Here's how the part is built. I have some questions about the finished solid (model axes, mm). Face numbers are marked on the shaded views. A direction names the side the tool comes from. Round coordinates to 2 decimals unless told otherwise and drop trailing zeros. Write each loop counter-clockwise with the first axis right and the second up, starting at its lowest first coordinate (ties: lowest second). Pieces come first, ordered by that corner, then holes. Notation, with made-up numbers: (3, 27.5) - (52, 27.5) arc R36 ccw to (52, 64.5) - close; hole circle Ø1 at (58, -15). An arc over 180 degrees is marked (long way). Write item = value, one per line. Start each with the question number.
Item 1: Thinking about a two-plate mould opening in Z: for the marked faces 3, 4 and 5, which applies, pulls with the +Z half, pulls with the -Z half, needs draft (parallel to the pull), parting line crosses it, or undercut?
Item 2: Which directions (+Z, -Z, +X, -X, +Y, -Y) give clear straight access to the entire face, cutting with the end or side of a thin tool? Please do the marked faces 1 and 2.
Item 3: If we section it at D-D (x = 64): Please give me the cut outline in (y, z), and give its area (3 significant figures).
Item 4: If we section it at A-A (y = 57): Please give me the cut outline in (x, z), and give its area (3 significant figures).
Item 5: For P1, Ø4, axis at x = -69.3, z = -81.8, coming from the +Y side; P2, Ø1.5, axis at x = -69.5, z = 81, coming from the -Y side; P3, Ø2, axis at x = 12, y = 74, coming from the +Z side, each with a flat end and sliding along its axis, tell me the tip position at first contact or that it passes through.
Item 6: If we section it at B-B (x = -69.3): Please give me the cut outline in (y, z).
Item 7: If I drill on line 1 along Z through (x, y) = (-69.3, 2); line 2 along X through (y, z) = (78, -24.5); line 3 along Z through (x, y) = (0, 63), over which ranges is the centre line in solid material (lowest first)? Write a range as [from, to].
Item 8: If we section it at C-C (z = -24.5): Please give me the cut outline in (x, y), and give its area (3 significant figures).
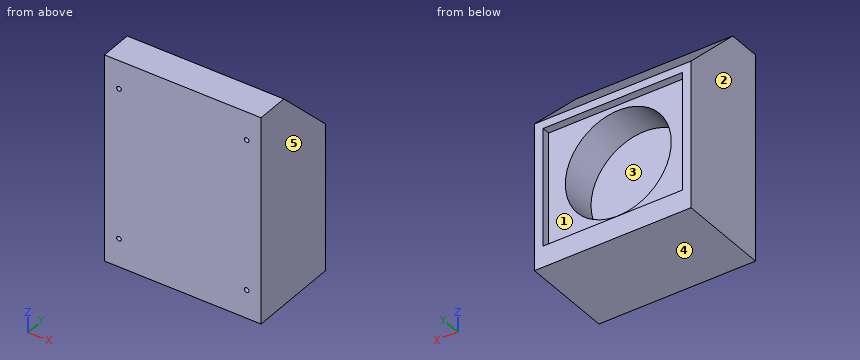
Autodesk Inventor part; units mm, degrees
ref_plane "YZ Plane" through (0, 0, 0) normal (1, 0, 0) x (0, 1, 0)
ref_plane "XZ Plane" through (0, 0, 0) normal (0, 1, 0) x (-1, 0, 0)
ref_plane "XY Plane" through (0, 0, 0) normal (0, 0, 1) x (1, 0, 0)
sketch "Sketch1" plane through (0, 0, 0) normal (0, 1, 0) x (-1, 0, 0)
  line L0 (-85, 112.5) -> (85, 112.5)
  line L1 (85, 112.5) -> (85, -112.5)
  line L2 (85, -112.5) -> (-85, -112.5)
  line L3 (-85, -112.5) -> (-85, 112.5)
  line L4 (-85, 112.5) -> (85, -112.5) construction
  line L5 (85, 112.5) -> (-85, -112.5) construction
  circle A0 centre (69.3, 81.8) radius 2.5
  circle A1 centre (69.3, -81.8) radius 2.5
  circle A2 centre (-69.3, -81.8) radius 2.5
  circle A3 centre (-69.3, 81.8) radius 2.5
  line L6 (69.3, 81.8) -> (-69.3, 81.8) construction
  line L7 (69.3, 81.8) -> (69.3, -81.8) construction
  line L8 (69.3, -81.8) -> (-69.3, -81.8) construction
  line L9 (69.3, 0) -> (0, 0) construction
  line L10 (0, 81.8) -> (0, 0) construction
  dimension "d2" = 170
  dimension "d3" = 225
  dimension "d9" = 163.6
  dimension "d10" = 5
  dimension "d11" = 138.6
extrude "Extrusion1" add sketch "Sketch1" along normal blind 100.5 contours L0 L1 L2 L3 | A0 | A1 | A2 | A3
extrude "Extrusion2" cut sketch "Sketch1" along normal blind 10 contours A0 | A1 | A2 | A3
chamfer "Chamfer1" distance 65 angle 45 1 edges at (0, 100.5, 112.5)
sketch "Sketch2" plane through (0, 100.5, 0) normal (0, 1, 0) x (1, 0, 0)
  line L0 (75.65, -38.8) -> (-75.65, -38.8)
  line L1 (-75.65, -38.8) -> (-75.65, 89.5)
  line L2 (-75.65, 89.5) -> (75.65, 89.5)
  line L3 (75.65, 89.5) -> (75.65, -38.8)
  line L4 (75.65, -38.8) -> (-75.65, 89.5) construction
  line L5 (-75.65, -38.8) -> (75.65, 89.5) construction
  line L6 (85, -47.5) -> (-85, -47.5)
  line L7 (85, -47.5) -> (85, 112.5)
  line L8 (85, 112.5) -> (-85, 112.5)
  line L9 (-85, 112.5) -> (-85, -47.5)
  line L10 (0, 89.5) -> (0, 112.5) construction
  circle A0 centre (0, 24.5) radius 57.5
  line L11 (0, 24.5) -> (0, 82) construction
  line L12 (0, 82) -> (0, 89.5) construction
  point P0 (0, 0)
  dimension "d21" = 115
  dimension "d18" = 151.3
  dimension "d19" = 128.3
  dimension "d20" = 23
  dimension "d22" = 7.5
extrude "Extrusion3" cut sketch "Sketch2" against normal blind 8.6 contours L0 L1 L2 L3 | A0
extrude "Extrusion4" cut sketch "Sketch2" against normal blind 40 from surface at -8.6 contours A0
properties part number "Spin Coater"
Reply:
q1.face_3 = undercut
q1.face_4 = pulls with the -Z half
q1.face_5 = needs draft
q2.face_1 = +Y
q2.face_2 = +Z, -Z, -X, +Y, -Y
q3.outline = (0, -112.5) - (100.5, -112.5) - (100.5, -89.5) - (91.9, -89.5) - (91.9, 38.8) - (100.5, 38.8) - (100.5, 47.5) - (35.5, 112.5) - (0, 112.5) - close
q3.area = 19,400 mm2
q4.outline = (-85, -112.5) - (85, -112.5) - (85, 91) - (-85, 91) - close; hole circle Ø115 at (0, -24.5)
q4.area = 24,200 mm2
q5.P1 = 91.9
q5.P2 = 10
q5.P3 = 75
q6.outline = (0, -112.5) - (100.5, -112.5) - (100.5, -89.5) - (91.9, -89.5) - (91.9, 38.8) - (100.5, 38.8) - (100.5, 47.5) - (35.5, 112.5) - (0, 112.5) - (0, 84.3) - (10, 84.3) - (10, 79.3) - (0, 79.3) - (0, -79.3) - (10, -79.3) - (10, -84.3) - (0, -84.3) - close
q7.line_1 = [-112.5, -84.3], [-79.3, 79.3], [84.3, 112.5]
q7.line_2 = [-85, -57.5], [57.5, 85]
q7.line_3 = [-112.5, -82], [33, 85]
q8.outline = (-85, 0) - (85, 0) - (85, 100.5) - (75.65, 100.5) - (75.65, 91.9) - (57.5, 91.9) - (57.5, 51.9) - (-57.5, 51.9) - (-57.5, 91.9) - (-75.65, 91.9) - (-75.65, 100.5) - (-85, 100.5) - close
q8.area = 11,200 mm2
